from build123d import *

# Parameters (mm, degrees)
SKETCH1_R               = 4
BOSS_EXTRUDE1_DEPTH     = 10
CUT_EXTRUDE2_DEPTH      = 72.414284285
CUT_EXTRUDE2_DEPTH_BACK = 72.414284285
SKETCH2_W               = 25
SKETCH2_H               = 5
HOLE1_D                 = 10
HOLE1_CBORE_D           = 18
HOLE1_CBORE_DEPTH       = 3


with BuildPart() as part:
    # Sketch1 → Boss-Extrude1 (new, symmetric)
    with BuildSketch(Plane.XY):
        with BuildLine():
            Line((0, 10), (60, 10))
            ThreePointArc((60, 10), (70, 0), (60, -10))
            Line((60, -10), (0, -10))
            ThreePointArc((0, -10), (-10, 0), (0, 10))
        make_face()
        Circle(SKETCH1_R, mode=Mode.SUBTRACT)
        with Locations((60, 0)):
            Circle(SKETCH1_R, mode=Mode.SUBTRACT)
    extrude(amount=BOSS_EXTRUDE1_DEPTH, both=True)

    # Sketch2 → Cut-Extrude2 (cut, two sides: drawn at the far end of the back side and taken through both)
    with BuildSketch(Plane(origin=(0, 0, 0), x_dir=(1, 0, 0), z_dir=(0, 1, 0)).offset(-CUT_EXTRUDE2_DEPTH_BACK)):
        with Locations((57.5, 0)):
            Rectangle(SKETCH2_W, SKETCH2_H)
        with Locations((2.5, 0)):
            Rectangle(SKETCH2_W, SKETCH2_H)
    extrude(amount=CUT_EXTRUDE2_DEPTH + CUT_EXTRUDE2_DEPTH_BACK, mode=Mode.SUBTRACT)

    # Hole1 (through all)
    with Locations(Plane(origin=(0, 10, 0), x_dir=(1, 0, 0), z_dir=(0, 1, 0))):
        with Locations((30, 0)):
            CounterBoreHole(HOLE1_D / 2, HOLE1_CBORE_D / 2, HOLE1_CBORE_DEPTH)


solid = part.part
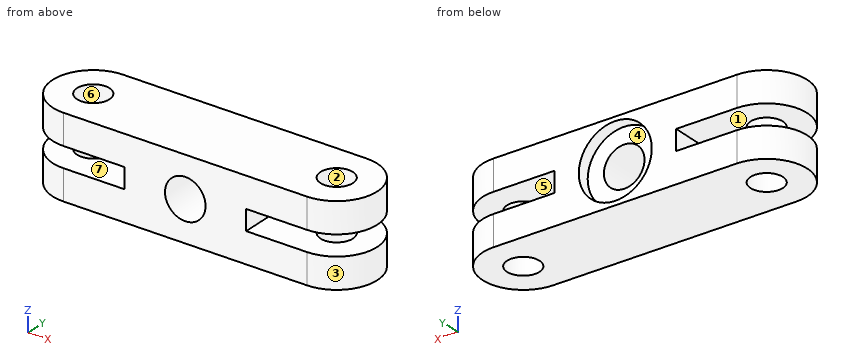
Geometry: final body of the model. Coordinates: model frame, mm. Face numbers are marked on the shaded views. A direction names the side the tool comes from. Give positions to 0.01 mm unless a question says otherwise; leave off trailing zeros. Order: outer loops, then holes, each group sorted by start corner. A loop starts at its lowest first (then second) coordinate and runs counter-clockwise, first axis right, second up. Notation, with made-up numbers: (85.25, 77.5) - (132.25, 77.5) arc R29 cw to (132.25, 101.5) - close; hole circle Ø1 at (23, 39). An arc over 180 degrees is marked (long way). Use CSV: the item, a comma, the result in double quotes.
1. Mould query, pull axis Y, two halves, no side actions, for the marked faces 1, 2 and 3. Classes: +Y half, -Y half, draft (parallel to the pull), parting line (faces both ways), or undercut.
Answers below:
face 1,"draft"
face 2,"undercut"
face 3,"parting line"
2. Contact query for flat-ended pins moving along their axis: pin 1 (5 mm diameter, centred on x = 0, y = 0, fed in from -Z) (3 decimals); pin 2 (1.5 mm diameter, centred on y = -0.5, z = 1, fed in from -X); pin 3 (5 mm diameter, centred on y = -4, z = 1, fed in from -X); pin 4 (5.5 mm diameter, centred on y = 4.5, z = 0.5, fed in from +X). Output: stop coordinate, or through.
Answers below:
pin 1,"through"
pin 2,"x = 15"
pin 3,"x = -9.8"
pin 4,"x = 69.65"
3. Section query A-A (y = 0). Give the number of separate pieces and of enclosed holes in the cut face, plus the area to 3 significant figures.
Answers below:
separate pieces,"5"
enclosed holes,"1"
area,"1,030 mm2"
4. Material intervals for line 1 along X through (y, z) = (0, -7.75); line 2 along Y through (x, z) = (60, 6.75); line 3 along Z through (x, y) = (30, 8.3), sorted ascending. Write a range as from..to.
Answers below:
line 1,"-10..-4, 4..56, 64..70"
line 2,"-10..-4, 4..10"
line 3,"-10..-9, 9..10"
5. Section query B-B (x = 47). Output: boundary loops of the cut face in (y, z), plus the area to 3 significant figures.
Answers below:
outline,"(-10, -10) - (10, -10) - (10, -2.5) - (-10, -2.5) - close; (-10, 2.5) - (10, 2.5) - (10, 10) - (-10, 10) - close"
area,"300 mm2"
6. Section query C-C (z = 0). Output: boundary loops of the cut face in (x, y), plus the area to 3 significant figures.
Answers below:
outline,"(15, -10) - (25, -10) - (25, 7) - (21, 7) - (21, 10) - (15, 10) - close; (35, -10) - (45, -10) - (45, 10) - (39, 10) - (39, 7) - (35, 7) - close"
area,"376 mm2"
7. Access query for the marked faces 4, 5, 6 and 7. Directions: +Z, -Z, +X, -X, +Y, -Y. A direction counts if a zero-diameter tool reaches every point of the face in a straight line with its end or side. Return the directions, or none.
Answers below:
face 4,"+Y"
face 5,"+X, +Y, -Y"
face 6,"+Z, -Z"
face 7,"-X, +Y, -Y"
8. Section query D-D (z = -4.25). Output: boundary loops of the cut face in (x, y).
Answers below:
outline,"(0, -10) - (27.37, -10) - (27.37, 7) - (22.07, 7) - (22.07, 10) - (0, 10) arc R10 ccw to start; (32.63, -10) - (60, -10) arc R10 ccw to (60, 10) - (37.93, 10) - (37.93, 7) - (32.63, 7) - close; hole circle Ø8 at (0, 0); hole circle Ø8 at (60, 0)"
